Build history of the part. All positions in model axes, mm. A direction names the side the tool comes from. Round coordinates to 2 decimals unless told otherwise and drop trailing zeros. Write each loop counter-clockwise with the first axis right and the second up, starting at its lowest first coordinate (ties: lowest second). Pieces come first, ordered by that corner, then holes. Notation, with made-up numbers: (4.5, 18.5) -> (24.5, 18.5) arc R15 ccw to (24.5, 36.5) -> close; hole circle Ø5 at (82.5, -34). An arc over 180 degrees is marked (long way). Return JSON: item names as keys, results as strings.
from build123d import *

# Parameters (mm, degrees)
F0_W     = 95
F0_H     = 95
F1_DEPTH = 30
F2_R     = 9
F3_DEPTH = 40
F4_W     = 66
F4_H     = 66
F5_DEPTH = 25.2
F6_R     = 11


with BuildPart() as f1:
    # F0 (on Front) → F1 (new body)
    with BuildSketch(Plane.XZ):
        Rectangle(F0_W, F0_H)
    extrude(amount=F1_DEPTH)

    # F2 (on face) → F3 (cut)
    with BuildSketch(Plane.XZ.offset(30)):
        with Locations((47.5, 47.5)):
            Circle(F2_R)
    extrude(amount=-F3_DEPTH, mode=Mode.SUBTRACT)

    # F4 (on face) → F5 (cut)
    with BuildSketch(Plane(origin=(0, 0, 0), x_dir=(-1, 0, 0), z_dir=(0, 1, 0))):
        with Locations((-47.5, 47.5)):
            Rectangle(F4_W, F4_H)
    extrude(amount=-F5_DEPTH, mode=Mode.SUBTRACT)

    # F6
    f6_edges = [f1.edges().sort_by_distance(p)[0] for p in [
        (14.5, -12.6, 14.5),
    ]]
    fillet(f6_edges, radius=F6_R)


solid = f1.part
Q1. Saw through at A-A on y = -3.75. List the corners of the cut face in (x, z), then the cut area to 3 significant figures.
Verdict:
{"outline": "(-47.5, -47.5) -> (47.5, -47.5) -> (47.5, 14.5) -> (25.5, 14.5) arc R11 cw to (14.5, 25.5) -> (14.5, 47.5) -> (-47.5, 47.5) -> close", "area": "7,960 mm²"}
Q2. Saw through at C-C on x = 32.5. List the corners of the cut face in (y, z).
Verdict:
{"outline": "(-30, -47.5) -> (0, -47.5) -> (0, 14.5) -> (-25.2, 14.5) -> (-25.2, 47.5) -> (-30, 47.5) -> close"}
Q3. Wall check: L1, parallel to Y at x = 30.5, z = 19.5; L2, parallel to X at y = -25, z = 30. Give the ranges that are in metal, low to high.
Verdict:
{"L1": "y = -30 to -25.2", "L2": "x = -47.5 to 14.5"}
Q4. Pin check, flat tips, straight feed: pin 1 Ø11 at (y, z) = (-7, 42) entering from +X; pin 2 Ø11 at (x, y) = (41, -7.5) entering from +Z. Stop position of each tip, or through.
Verdict:
{"pin 1": "stops at x = 14.5", "pin 2": "stops at z = 14.5"}
Q5. Saw through at B-B on z = 35. List the corners of the cut face in (x, y), then the cut area to 3 significant figures.
Verdict:
{"outline": "(-47.5, -30) -> (47.5, -30) -> (47.5, -25.2) -> (14.5, -25.2) -> (14.5, 0) -> (-47.5, 0) -> close", "area": "2,020 mm²"}
Q6. 3-axis set-ups, long thin cutter, end or side, ignore diameter. For faces 1 (the flat face through (37, -12, 14.5)), 2 (the cylindrical face through (41.066, -27.634, 41.206)): which of +Z, -Z, +X, -X, +Y, -Y reach the whole face in a straight line?
Verdict:
{"face 1": "+Z, +X, +Y", "face 2": "+Z, +X, +Y, -Y"}
